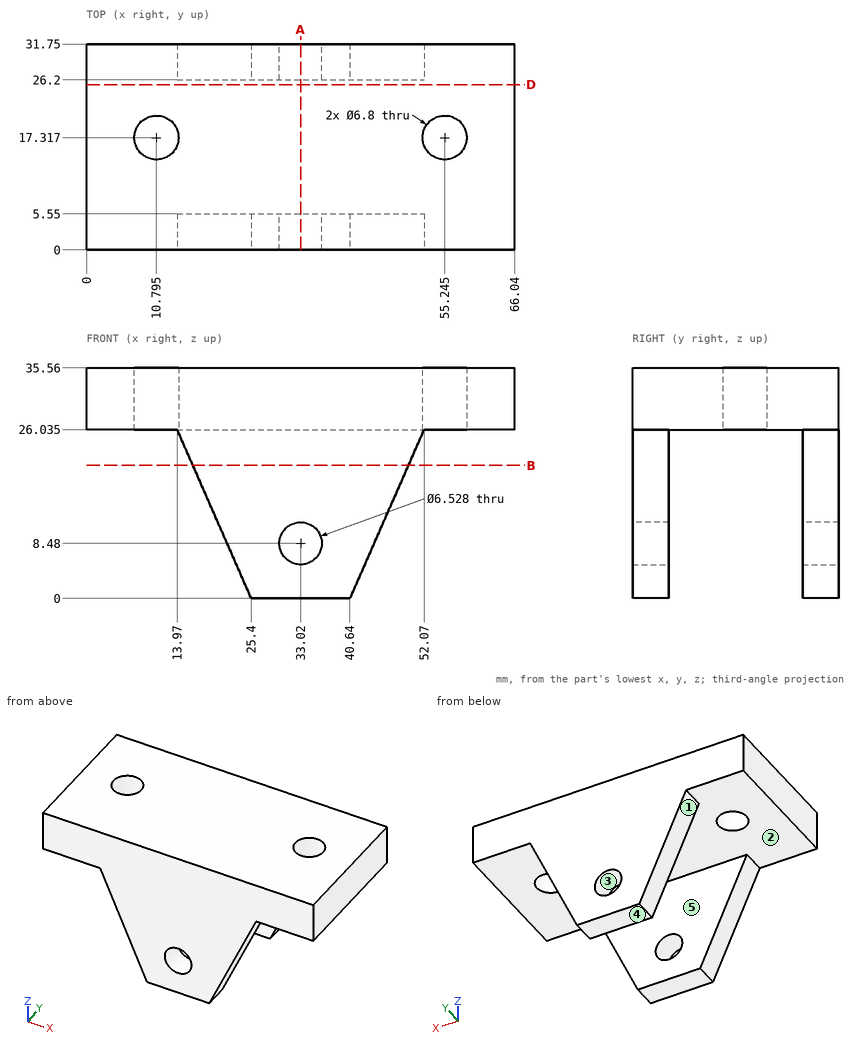
The figure shows three views and two pictorial views of one solid part (mm, origin at its lowest corner). Answer the questions. A direction names the side the tool comes from. Coordinates: 2 decimals unless noted, no trailing zeros. Write each loop counter-clockwise with the first axis right and the second up, starting at its lowest first coordinate (ties: lowest second). Pieces come first, ordered by that corner, then holes.
1. The part is cut by section A-A, the plane x = 33.02. State how many separate pieces and enclosed holes the cut face has, and give its area (3 significant figures).
Results list:
separate pieces: 3
enclosed holes: 0
area: 519 mm2
2. Flat-ended cylindrical pins translate along their axes: pin 1 (8 mm diameter, centred on x = 33, z = 17, fed in from -Y); pin 2 (3 mm diameter, centred on y = 26, z = 11.5, fed in from +X); pin 3 (1.5 mm diameter, centred on x = 44, y = 16.5, fed in from -Z) (3 decimals); pin 4 (5 mm diameter, centred on x = 33.02, z = 8.48, fed in from -Y). Find the tip coordinate at first contact, or state that the pin passes through.
Results list:
pin 1: stops at y = 0
pin 2: stops at x = 46.34
pin 3: stops at z = 26.035
pin 4: passes through
3. The part is cut by section B-B, the plane z = 20.5. Write down the section's boundary in (x, y).
Results list:
outline: (16.4, 0) - (49.64, 0) - (49.64, 5.55) - (16.4, 5.55) - close; (16.4, 26.2) - (49.64, 26.2) - (49.64, 31.75) - (16.4, 31.75) - close
4. The part is cut by section D-D, the plane y = 25.5. Write down the section's boundary in (x, z) (1 decimal), and give its area (3 significant figures).
Results list:
outline: (0, 26) - (66, 26) - (66, 35.6) - (0, 35.6) - close
area: 629 mm2
5. Consider line 1 along Z through (x, y) = (33, 4); line 2 along Y through (x, z) = (35, 19.5); line 3 along Z through (x, y) = (6.5, 18) (1 decimal). Determine where each line is inside the solid, lowest interval first.
Results list:
line 1: z = 0 to 5.22, 11.74 to 35.56
line 2: y = 0 to 5.55, 26.2 to 31.75
line 3: z = 26 to 35.6
6. For a pull along Z with two mould halves and no side action, classify the marked faces 3, 4 and 5 as +Z half, -Z half, draft (parallel to the pull), parting line (faces both ways), or undercut.
Results list:
face 3: undercut
face 4: -Z half
face 5: draft
7. For the marked faces 1 and 2, determine the directions among +Z, -Z, +X, -X, +Y, -Y from which every point of the face is accessible in a straight line to the end or side of a thin tool.
Results list:
face 1: -Z, -X, +Y, -Y
face 2: -Z
